Autodesk Inventor part; units mm, degrees
ref_plane "YZ Plane" through (0, 0, 0) normal (1, 0, 0) x (0, 1, 0)
ref_plane "XZ Plane" through (0, 0, 0) normal (0, 1, 0) x (-1, 0, 0)
ref_plane "XY Plane" through (0, 0, 0) normal (0, 0, 1) x (1, 0, 0)
sketch "Sketch1" plane through (0, 0, 0) normal (0, 1, 0) x (-1, 0, 0)
  line L0 (0, 0) -> (0, 71)
  line L1 (0, 71) -> (-5, 71)
  line L2 (-5, 71) -> (-20, 0)
  line L3 (-20, 0) -> (0, 0)
  dimension "d0" = 71
  dimension "d1" = 20
  dimension "d2" = 5
extrude "Extrusion1" add sketch "Sketch1" along normal blind 55
sketch "Sketch2" plane through (0, 0, 0) normal (-1, 0, 0) x (0, 0, 1)
  circle A0 centre (23, 22.6) radius 2.55
  circle A1 centre (58, 22.6) radius 2.55
  circle A2 centre (40.5, 15) radius 2.55
  line L0 (23, 22.6) -> (58, 22.6) construction
  line L1 (40.5, 22.6) -> (40.5, 15) construction
  line L2 (71, 0) -> (71, 55) construction
  point P0 (0, 0)
  dimension "d5" = 5.1
  dimension "d6" = 35
  dimension "d7" = 7.6
  dimension "d8" = 15
  dimension "d9" = 30.5
extrude "Extrusion2" cut sketch "Sketch2" against normal blind 45
sketch "Sketch3" plane through (20, 0, 0) normal (0, 0, -1) x (-1, 0, 0)
  line L0 (0, 0) -> (0, 55)
  line L1 (0, 51.5) -> (10, 51.5)
  arc A0 (15, 46.5) -> (10, 51.5) centre (10, 46.5) ccw
  line L2 (15, 46.5) -> (15, 8.5)
  arc A1 (10, 3.5) -> (15, 8.5) centre (10, 8.5) ccw
  line L3 (10, 3.5) -> (0, 3.5)
  line L4 (15, 27.5) -> (0, 27.5) construction
  point P0 (20, 0)
  dimension "d12" = 3.5
  dimension "d13" = 3.5
  dimension "d14" = 5
  dimension "d15" = 5
extrude "Extrusion3" cut sketch "Sketch3" against normal through all
sketch "Sketch5" plane through (20, 0, 0) normal (0, 0, -1) x (-1, 0, 0)
  line L0 (20, 0) -> (20, 55)
  line L1 (0, 55) -> (20, 55)
  line L2 (0, 0) -> (20, 0)
  line L3 (0, 51.5) -> (0, 55)
  line L4 (0, 55) -> (0, 0)
extrude "Extrusion4" add sketch "Sketch5" along normal blind 3.5
sketch "Sketch6" plane through (20, 0, 0) normal (0, 0, 1) x (1, 0, 0)
  circle A0 centre (-8, 12.5) radius 2.54
  circle A1 centre (-8, 42.5) radius 2.54
  line L0 (-8, 12.5) -> (-8, 42.5) construction
  line L1 (-20, 0) -> (-20, 55)
  line L2 (-20, 27.5) -> (-8, 27.5) construction
  line L3 (-15, 8.5) -> (-15, 46.5) construction
  line L4 (0, 51.5) -> (0, 3.5) construction
  line L5 (-15, 46.5) -> (-15, 8.5)
  line L6 (-15, 12.5) -> (-8, 12.5) construction
  line L7 (-8, 12.5) -> (0, 12.5) construction
  dimension "d20" = 5.08
  dimension "d21" = 30
  dimension "d22" = 8
extrude "Extrusion5" cut sketch "Sketch6" against normal through all
fillet "Fillet1" radius 3 5 edges at (6.4645, 4.9645, 0) (15, 3.5, 0) (6.4645, 50.0355, 0) (15, 51.5, 0) (5, 27.5, 0)
fillet "Fillet2" radius 3 2 edges at (12.5, 0, 35.5) (12.5, 55, 35.5)
properties part number "Cable_Chain_Side_Holder"
Design review of the part built by this model. Coordinates are the model's own, in mm. A direction names the side the tool comes from. Coordinates: 2 decimals unless noted, no trailing zeros. Order: outer loops, then holes, each group sorted by start corner. A loop starts at its lowest first (then second) coordinate and runs counter-clockwise, first axis right, second up. Notation, with made-up numbers: M 3,-30 L 33,-30 A17 ccw 33,-2 Z; hole C 17.25,20.5 d2. An arc over 180 degrees is marked long. Answer as a JSON object with one key per item and string values. Group by question number.
1) Mouldability with a two-part tool opening along Y and no side actions: class faces 1 (the cylindrical face through (12.06, 0.9, 33.43)), 2 (the cylindrical face through (14.93, 4.4, 0.86)), 3 (the flat face through (0, 27, 34)) as pulls with the +Y half, pulls with the -Y half, needs draft (parallel to the pull), parting line crosses it, or undercut.
2) Add section D-D, the plane y = 16.5. Write out the cut boundary in (x, z), then the cut area to 3 significant figures.
3) For pin 1 (8 mm diameter, centred on x = 12, y = 12.5, fed in from -Z); pin 2 (10 mm diameter, centred on x = 14, y = 39.5, fed in from +Z); pin 3 (3 mm diameter, centred on x = 14, z = 29, fed in from -Y), all flat-tipped, find the tip position at first contact; note any pin that passes through.
4) Wall thickness on L1, parallel to Y at x = 12, z = -2.2; L2, parallel to Y at x = 3.4, z = 40.5; L3, parallel to Y at x = 3.2, z = 23: over which ranges is each line inside the solid? List them lowest first.
5) Tool access review of faces 4 (the cylindrical face through (15.07, 50.6, 0.86)), 5 (the cylindrical face through (10.13, 44.22, -1.73)): name each direction out of +Z, -Z, +X, -X, +Y, -Y from which nothing blocks a thin tool from reaching the whole face with its end or side.
6) Add section C-C, the plane x = 3.5. Count the separate pieces of the cut face and the enclosed holes in it, then the cut area to 3 significant figures.
7) Add section B-B, the plane y = 36.5. Write out the cut boundary in (x, z).
8) Add section A-A, the plane y = 42.5. Write out the cut boundary in (x, z), then the cut area to 3 significant figures.
Computed values:
{
 "1": {"face 1": "pulls with the -Y half", "face 2": "undercut", "face 3": "needs draft"},
 "2": {"outline": "M 0,-3.5 L 20,-3.5 L 20,0 L 8,0 A3 cw 5,3 L 5,38.44 L 0,38.44 Z; M 0,42.56 L 5,42.56 L 5,71 L 0,71 Z", "area": "406 mm^2"},
 "3": {"pin 1": "stops at z = -3.5", "pin 2": "stops at z = 0", "pin 3": "stops at y = 0.48"},
 "4": {"L1": "y = 0 to 9.96, 15.04 to 39.96, 45.04 to 55", "L2": "y = 0 to 12.45, 17.55 to 55", "L3": "y = 0 to 20.05, 25.15 to 55"},
 "5": {"face 4": "+Z, +X", "face 5": "+Z, -Z"},
 "6": {"separate pieces": "1", "enclosed holes": "3", "area": "4,030 mm^2"},
 "7": {"outline": "M 0,-3.5 L 20,-3.5 L 20,0 L 8,0 A3 cw 5,3 L 5,71 L 0,71 Z"},
 "8": {"outline": "M 0,-3.5 L 9.46,-3.5 L 9.46,0 L 8,0 A3 cw 5,3 L 5,71 L 0,71 Z; M 14.54,-3.5 L 20,-3.5 L 20,0 L 14.54,0 Z", "area": "409 mm^2"}
}
